from build123d import *


with BuildPart() as f1:
    # F0 (on Front) → F1 (revolve)
    with BuildSketch(Plane.XZ):
        with BuildLine():
            Line((4.338621, 3), (15, 3))
            Line((15, 3), (15, 7))
            Line((15, 7), (7, 7))
            Line((7, 7), (7, 10))
            Line((7, 10), (15, 10))
            Line((15, 10), (15, 13))
            Line((15, 13), (0.029517, 13.095834))
            Line((0.029517, 13.095834), (0.848745, 11.908195))
            ThreePointArc((0.848745, 11.908195), (1.506784, 10.555919), (1.732951, 9.069139))
            Line((1.732951, 9.069139), (1.732951, 7.126357))
            ThreePointArc((1.732951, 7.126357), (1.365156, 4.439235), (0.288825, 1.949774))
            ThreePointArc((0.288825, 1.949774), (0.073559, 1.451882), (0, 0.914457))
            Line((0, 0.914457), (0, 0))
            Line((0, 0), (4.338621, 0))
            Line((4.338621, 0), (4.338621, 3))
        make_face()
    revolve(axis=Axis((8.018091, 0, 0), (1, 0, 0)))


solid = f1.part
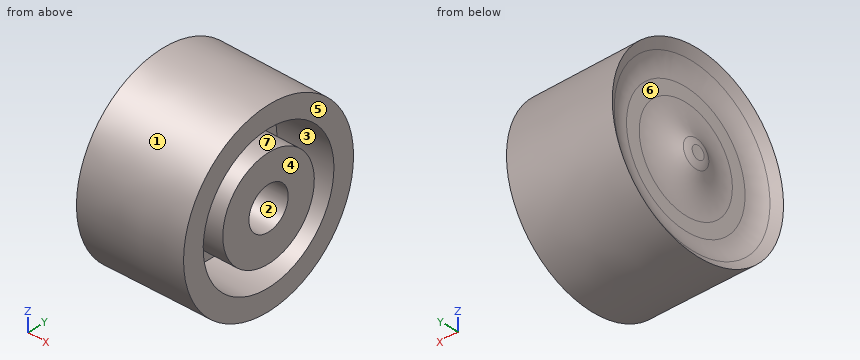
For this review, take the finished solid that the model builds, in its own axes (mm). Face numbers are marked on the shaded views. A direction names the side the tool comes from. Round coordinates to 2 decimals unless told otherwise and drop trailing zeros. Write each loop counter-clockwise with the first axis right and the second up, starting at its lowest first coordinate (ties: lowest second). Pieces come first, ordered by that corner, then holes. Notation, with made-up numbers: (5.5, 67) -> (49.5, 67) arc R12 cw to (49.5, 78) -> close; hole circle Ø6 at (63.25, -19). An arc over 180 degrees is marked (long way). Use CSV: the item, a comma, the result in double quotes.
(1) Clearance check with flat-ended pins moving along their axes: P1, Ø3, axis at x = 8.5, z = 0.5, coming from the -Y side; P2, Ø4, axis at y = -8.5, z = -5.5, coming from the -X side; P3, Ø1, axis at x = 10, y = -3.5, coming from the +Z side. State where each tip first meets the part, or that it passes through.
Computed values:
P1,"y = -13.05"
P2,"x = 0.7"
P3,"z = 12.68"
(2) For the marked faces 5, 6 and 7, list the 3-axis set-ups (+Z, -Z, +X, -X, +Y, -Y) from which the entire face can be reached by the end or side of a thin tool; tool diameter is ignored.
Computed values:
face 5,"+Z, -Z, +X, +Y, -Y"
face 6,"-X"
face 7,"+X"
(3) Consider section B-B, the plane x = 3.5. Give the boundary of the cut face in (y, z).
Computed values:
outline,"circle Ø26.15 at (0, 0)"
(4) Draft analysis for pull direction Z (two halves, no side actions). For the marked faces 1, 2, 3 and 4, state which applies: +Z half, -Z half, draft (parallel to the pull), parting line (faces both ways), or undercut.
Computed values:
face 1,"parting line"
face 2,"undercut"
face 3,"undercut"
face 4,"draft"
(5) Consider section A-A, the plane x = 13.5. Give the boundary of the cut face in (y, z).
Computed values:
outline,"circle Ø26.02 at (0, 0); circle Ø14 at (0, 0); hole circle Ø20 at (0, 0); hole circle Ø6 at (0, 0)"
(6) To check wall thickness, follow L1, parallel to Y at x = 13, z = 0; L2, parallel to Y at x = 7.25, z = -6; L3, parallel to Z at x = 8.75, y = 0. State the ranges of each line that lie inside material, in increasing order. Write a range as [from, to].
Computed values:
L1,"[-13.01, -10], [-7, -3], [3, 7], [10, 13.01]"
L2,"[-11.59, -8], [-3.61, 3.61], [8, 11.59]"
L3,"[-13.04, -10], [-7, -3], [3, 7], [10, 13.04]"
